Autodesk Inventor part; units mm, degrees
ref_plane "YZ Plane" through (0, 0, 0) normal (1, 0, 0) x (0, 1, 0)
ref_plane "XZ Plane" through (0, 0, 0) normal (0, 1, 0) x (-1, 0, 0)
ref_plane "XY Plane" through (0, 0, 0) normal (0, 0, 1) x (1, 0, 0)
sketch "Sketch1" plane through (0, 0, 0) normal (0, 0, 1) x (1, 0, 0)
  spline S0 degree 3 poles (5, 2.8134) (4.7282, 2.7718) (4.4577, 2.7171) (3.9725, 2.5829) (3.7572, 2.5096) (3.2649, 2.2994) (2.9924, 2.1483) (2.5895, 1.8431) (2.4453, 1.712) (2.3168, 1.5682) (2.1311, 1.3604) (1.976, 1.1232) (1.7525, 0.5925) (1.6905, 0.2977) (1.6905, 0) knots 0 0 0 0 0.174284 0.174284 0.317468 0.317468 0.513399 0.513399 0.635856 0.635856 0.635856 0.812785 0.812785 1 1 1 1
  line L0 (5, 2.8134) -> (5, 10)
  line L1 (0, 10) -> (5, 10)
  line L2 (0, 2.607) -> (0, 10)
  spline S1 degree 3 poles (1.5054, -1.0718) (1.0443, -0.6134) (0.6771, -0.0703) (0.2854, 0.8445) (0.1821, 1.1739) (0.0367, 1.8715) (0, 2.2339) (0, 2.607) knots 0 0 0 0 0.47732 0.47732 0.730106 0.730106 1 1 1 1
  spline S2 degree 3 poles (1.6905, -1.2645) (1.6303, -1.1989) (1.5686, -1.1346) (1.5054, -1.0718) knots 0 0 0 0 1 1 1 1
  line L3 (1.6905, 0) -> (1.6905, -1.2645)
  circle A0 centre (2.5, 7) radius 1
  circle A1 centre (12.5, 7) radius 1
  spline S3 degree 3 poles (13.3095, 0) (13.3095, 0.2448) (13.2668, 0.4921) (13.0809, 1.0308) (12.9041, 1.3201) (12.6871, 1.5639) (12.5591, 1.7077) (12.4154, 1.8388) (12.0138, 2.1444) (11.7421, 2.2958) (11.2512, 2.5065) (11.0368, 2.5799) (10.5491, 2.7158) (10.2752, 2.7712) (10, 2.8134) knots 0 0 0 0 0.154789 0.154789 0.362213 0.362213 0.362213 0.4846 0.4846 0.68042 0.68042 0.823311 0.823311 1 1 1 1
  line L4 (13.3095, -1.2645) -> (13.3095, 0)
  spline S4 degree 3 poles (13.3095, -1.2645) (13.3697, -1.1989) (13.4314, -1.1346) (13.4946, -1.0718) knots 0 0 0 0 1 1 1 1
  spline S5 degree 3 poles (15, 2.607) (15, 2.4473) (14.9933, 2.2901) (14.9258, 1.5152) (14.7659, 0.9156) (14.2513, -0.1742) (13.9111, -0.6578) (13.4946, -1.0718) knots 0 0 0 0 0.115959 0.115959 0.56908 0.56908 1 1 1 1
  line L5 (15, 2.607) -> (15, 10)
  line L6 (10, 10) -> (15, 10)
  line L7 (10, 10) -> (10, 2.8134)
  line L8 (0, 10) -> (15, 10)
  line L9 (15, 10) -> (15, 4)
  line L10 (15, 4) -> (0, 4)
  line L11 (0, 4) -> (0, 10)
  point P0 (0, 0)
  dimension "d0" = 15
  dimension "d1" = 6
extrude "Extrusion1" add sketch "Sketch1" along normal blind 4 contours L10 L2 L1 L0 | L0 L8 L7 L10 | L7 L6 L5 L10
sketch "Sketch2" plane through (0, 10, 0) normal (0, 1, 0) x (1, 0, 0)
  line L0 (15, 0) -> (0, 0)
  line L1 (0, 0) -> (0, -4)
  line L2 (15, -4) -> (0, -4)
  line L3 (15, 0) -> (15, -4)
  line L4 (15, -4) -> (0, -4)
  line L5 (0, -4) -> (15, -4)
  line L6 (15, -4) -> (15, 5)
  line L7 (15, 5) -> (0, 5)
  line L8 (0, 5) -> (0, -4)
  dimension "d4" = 15
  dimension "d5" = 9
extrude "Extrusion2" add sketch "Sketch2" along normal blind 80
sketch "Sketch3" plane through (15, 10, -5) normal (0, 0, -1) x (-1, 0, 0)
  line L0 (0, 0) -> (15, 0)
  line L1 (15, 0) -> (15, 80)
  line L2 (0, 80) -> (15, 80)
  line L3 (0, 0) -> (0, 80)
  line L4 (7.5, 80) -> (7.5, 38)
  line L5 (7.5, 18) -> (7.5, 58) construction
  line L6 (10.5, 18) -> (10.5, 58)
  line L7 (4.5, 58) -> (4.5, 18)
  arc A0 (4.5, 18) -> (10.5, 18) centre (7.5, 18) ccw
  arc A1 (10.5, 58) -> (4.5, 58) centre (7.5, 58) ccw
  point P0 (15, -10)
  dimension "d8" = 42
  dimension "d9" = 20
  dimension "d10" = 6
extrude "Extrusion3" cut sketch "Sketch3" against normal blind 80 contours A0 L7 A1 L6
chamfer "Chamfer1" distance 2 angle 45 4 edges at (15, 47, 4) (15, 50, -5) (0, 50, -5) (0, 47, 4)
chamfer "Chamfer2" distance 2 angle 45 1 edges at (7.5, 4, 4)
fillet "Fillet1" radius 2 4 edges at (1, 90, -4) (14, 90, -4) (14, 90, 3) (1, 90, 3)
properties part number "pen_2"
Geometry check sheet. Reference: the model listing, model coordinates, mm. A direction names the side the tool comes from. Coordinates: 2 decimals unless noted, no trailing zeros. Order: outer loops, then holes, each group sorted by start corner. A loop starts at its lowest first (then second) coordinate and runs counter-clockwise, first axis right, second up. Notation, with made-up numbers: (-27.75, 7.25) - (-21.75, 7.25) arc R22 ccw to (-21.75, 31.25) - close; hole circle Ø6 at (32, 52). An arc over 180 degrees is marked (long way). Answer in a Markdown table with one row per item. Add a question column.
1. Gauge pin test, flat ends, axial feed: pin 1 Ø1.5 at (x, z) = (10, -2.5) entering from -Y; pin 2 Ø3 at (x, y) = (5, 7) entering from -Z. Record the tip position at first contact, or that the pin passes through.
2. Section check D-D (z = 2.75). Give the number of separate pieces and of enclosed holes in the cut face, plus the area to 3 significant figures.
3. Draft check along Y on faces 4 (the face through (1.73, 89.65, 2.5)), 5 (the face through (4, 49, 4)), 6 (the face through (3.454, 6.7, 1.972)). Enter one of: +Y half, -Y half, draft (parallel to the pull), parting line (faces both ways), or undercut.
4. Section check B-B (y = 32.5). Enter the section's corners in (x, z), plus the area to 3 significant figures.
5. Access from +Z, -Z, +X, -X, +Y, -Y to the whole of each face (thin tool, end or side, straight path). Record for faces 1 (the face through (4.5, 48, -1)), 2 (the face through (7, 90, -1)), 3 (the face through (7, 10, -3)).
6. Material ranges on L1, parallel to X at y = 42.5, z = -2; L2, parallel to Y at x = 8.75, z = -3.5; L3, parallel to Y at x = 12.5, z = 2.9, recorded low to high. Write a range as [from, to].
7. Section check A-A (x = 7.5). Enter the section's corners in (y, z).
8. Section check C-C (y = 21.5). Enter the section's corners in (x, z), plus the area to 3 significant figures.
Data:
| question | item | result |
|---|---|---|
| 1 | pin 1 | stops at y = 10 |
| 1 | pin 2 | stops at z = 0 |
| 2 | separate pieces | 1 |
| 2 | enclosed holes | 3 |
| 2 | area | 874 mm² |
| 3 | face 4 | +Y half |
| 3 | face 5 | draft |
| 3 | face 6 | undercut |
| 4 | outline | (0, -3) - (2, -5) - (4.5, -5) - (4.5, 4) - (2, 4) - (0, 2) - close; (10.5, -5) - (13, -5) - (15, -3) - (15, 2) - (13, 4) - (10.5, 4) - close |
| 4 | area | 73.0 mm² |
| 5 | face 1 | +Z, -Z |
| 5 | face 2 | +Z, -Z, +X, -X, +Y |
| 5 | face 3 | -Z, +X, -X, -Y |
| 6 | L1 | x = [0, 4.5], [10.5, 15] |
| 6 | L2 | y = [10, 25.27], [70.73, 90] |
| 6 | L3 | y = [4.9, 6], [8, 89.8] |
| 7 | outline | (4, 0) - (10, 0) - (10, -5) - (25, -5) - (25, 4) - (6, 4) - (4, 2) - close; (71, -5) - (90, -5) - (90, 4) - (71, 4) - close |
| 8 | outline | (0, -3) - (2, -5) - (13, -5) - (15, -3) - (15, 2) - (13, 4) - (2, 4) - (0, 2) - close |
| 8 | area | 127 mm² |
